Autodesk Inventor part; units mm, degrees
ref_plane "IP_1_XY" through (0, 0, 0) normal (1, 0, 0) x (0, 0, -1)
ref_plane "IP_1_YZ" through (0, 0, 0) normal (0, 0, -1) x (0, 1, 0)
ref_plane "IP_1_ZX" through (0, 0, 0) normal (0, 1, 0) x (1, 0, 0)
sketch "Sketch_1" plane through (0, 0, 0) normal (0, 0, 1) x (1, 0, 0)
  line L0 (8, 0) -> (0, 0)
  line L1 (0, 2.1) -> (0.5, 2.1)
  line L2 (0.5, 2.1) -> (0.5, 3.2)
  arc A0 (0.8, 3.5) -> (0.5, 3.2) centre (0.8, 3.2) ccw
  line L3 (0.8, 3.5) -> (7.2, 3.5)
  arc A1 (7.5, 3.2) -> (7.2, 3.5) centre (7.2, 3.2) ccw
  line L4 (7.5, 3.2) -> (7.5, 2.1)
  line L5 (7.5, 2.1) -> (8, 2.1)
  line L6 (8, 2.1) -> (8, 3.2)
  arc A2 (8, 3.2) -> (7.2, 4) centre (7.2, 3.2) ccw
  line L7 (7.2, 4) -> (0.8, 4)
  arc A3 (0.8, 4) -> (0, 3.2) centre (0.8, 3.2) ccw
  line L8 (0, 3.2) -> (0, 2.1)
revolve "Revolution1" add sketch "Sketch_1" angle 360 about axis through (8, 0, 0) along (1, 0, 0)
ref_plane "IP_1_XY" through (0, 0, 0) normal (1, 0, 0) x (0, 0, -1)
ref_plane "IP_1_YZ" through (0, 0, 0) normal (0, 0, -1) x (0, 1, 0)
ref_plane "IP_1_ZX" through (0, 0, 0) normal (0, 1, 0) x (1, 0, 0)
ref_plane "IP_5_XY" through (4, 0, 0) normal (1, 0, 0) x (0, 0, -1)
ref_plane "IP_5_YZ" through (4, 0, 0) normal (0, 0, -1) x (0, 1, 0)
ref_plane "IP_5_ZX" through (4, 0, 0) normal (0, 1, 0) x (1, 0, 0)
ref_plane "IP_6_XY" through (5.6, 0, 0) normal (1, 0, 0) x (0, 0, -1)
ref_plane "IP_6_YZ" through (5.6, 0, 0) normal (0, 0, -1) x (0, 1, 0)
ref_plane "IP_6_ZX" through (5.6, 0, 0) normal (0, 1, 0) x (1, 0, 0)
properties part number "HK0408FT2SH"
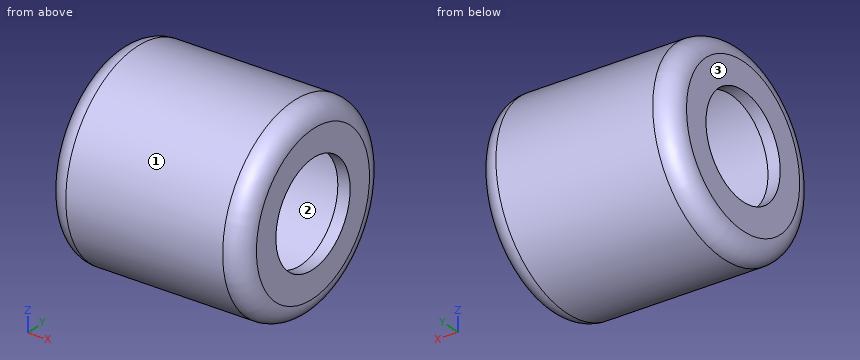
Could you check a few things on this model? Use its own coordinates, in mm. Face numbers are marked on the shaded views. Coordinates: 2 decimals unless noted, no trailing zeros. Loops run counter-clockwise (first coordinate to the right, second up) from the corner with the lowest first, then second, coordinate; pieces in that order, holes last. Notation, with made-up numbers: M 17.5,12 L 63.5,12 A14 ccw 63.5,32 Z; hole C 4,-36.75 d2. An arc over 180 degrees is marked long. Put each result on its own line as item: value. Start each with the question number.
(1) Suppose I cut it at C-C on x = 7. Please give me the cut outline in (y, z).
(2) Will these pins go through, and if not, where does the flat tip stop? P1, Ø3, axis at y = -0.5, z = -0.5, coming from the +X side; P2, Ø3, axis at x = 6, y = -2, coming from the -Z side; P3, Ø3.5, axis at y = 0, z = 0, coming from the +X side; P4, Ø4, axis at x = 3.5, z = -2.5, coming from the -Y side.
(3) Thinking about a two-plate mould opening in Z: for the marked faces 1, 2 and 3, which applies, pulls with the +Z half, pulls with the -Z half, needs draft (parallel to the pull), parting line crosses it, or undercut?
(4) Suppose I cut it at A-A on y = 0. Please give me the cut outline in (x, z), then the cut area to 3 significant figures.
(5) I need wall thicknesses on line 1 (X direction, y = 0.5, z = 2.5); line 2 (Z direction, x = 5.5, y = 1); line 3 (Y direction, x = 7, z = -2). Which ranges of each line are inside material? Lowest first, please. Write a range as from..to.
Solutions:
1. outline: C 0,0 d8; hole C 0,0 d7
2. P1: stops at x = 8
2. P2: stops at z = -3.97
2. P3: passes through
2. P4: stops at y = -3.97
3. face 1: parting line crosses it
3. face 2: undercut
3. face 3: needs draft
4. outline: M 0,-3.2 A0.8 ccw 0.8,-4 L 7.2,-4 A0.8 ccw 8,-3.2 L 8,-2.1 L 7.5,-2.1 L 7.5,-3.2 A0.3 cw 7.2,-3.5 L 0.8,-3.5 A0.3 cw 0.5,-3.2 L 0.5,-2.1 L 0,-2.1 Z; M 0,2.1 L 0.5,2.1 L 0.5,3.2 A0.3 cw 0.8,3.5 L 7.2,3.5 A0.3 cw 7.5,3.2 L 7.5,2.1 L 8,2.1 L 8,3.2 A0.8 ccw 7.2,4 L 0.8,4 A0.8 ccw 0,3.2 Z
4. area: 10.3 mm2
5. line 1: x = 0..0.5, 7.5..8
5. line 2: z = -3.87..-3.35, 3.35..3.87
5. line 3: y = -3.46..-2.87, 2.87..3.46
